from build123d import *

# Parameters (mm, degrees)
PAD023_DEPTH    = 13
SKETCH050_R     = 0.85
POCKET025_DEPTH = 5
FILLET008_R     = 1.2
SKETCH061_W     = 3.59
SKETCH061_H     = 1.95
PAD032_DEPTH    = 1.5
FILLET011_R     = 1


with BuildPart() as part:
    # Sketch049 → Pad023 (new body)
    with BuildSketch(Plane.XZ.offset(-4)):
        Polygon((24.862594, 8.175321), (27.662594, 8.175321), (27.662594, 7.975321), (31.362594, 7.975321), (31.362594, 6.775321), (24.862594, 6.775321), align=None)
    extrude(amount=PAD023_DEPTH)

    # Sketch050 (on Face5 of Pad023) → Pocket025 (cut)
    with BuildSketch(Plane(origin=(0, 0, 6.775321), x_dir=(1, 0, 0), z_dir=(0, 0, -1))):
        with Locations((29.62, 4.4)):
            Circle(SKETCH050_R)
        with Locations((29.62, 0.4)):
            Circle(SKETCH050_R)
    extrude(amount=-POCKET025_DEPTH, mode=Mode.SUBTRACT)

    # Fillet008
    fillet008_edges = [part.edges().sort_by_distance(p)[0] for p in [
        (24.862594, -9, 7.475321),
        (24.862594, 4, 7.475321),
    ]]
    fillet(fillet008_edges, radius=FILLET008_R)

    # Sketch061 (on Face9 of Fillet008) → Pad032 (join)
    with BuildSketch(Plane(origin=(0, 0, 7.975321), x_dir=(-1, 0, 0), z_dir=(0, 0, 1))):
        with Locations((-29.547098, 7.987892)):
            Rectangle(SKETCH061_W, SKETCH061_H)
        with Locations((-29.547098, -2.962108)):
            Rectangle(SKETCH061_W, SKETCH061_H)
    extrude(amount=PAD032_DEPTH)

    # Fillet011
    fillet011_edges = [part.edges().sort_by_distance(p)[0] for p in [
        (27.752098, 2.962108, 9.475321),
        (31.342098, 2.962108, 9.475321),
        (27.752098, -7.987892, 9.475321),
        (31.342098, -7.987892, 9.475321),
    ]]
    fillet(fillet011_edges, radius=FILLET011_R)


with BuildPart() as part_1:
    # Body006 placement: moved
    add(part.part.moved(Location((0, -8.6, 0.6))))


solid = part_1.part
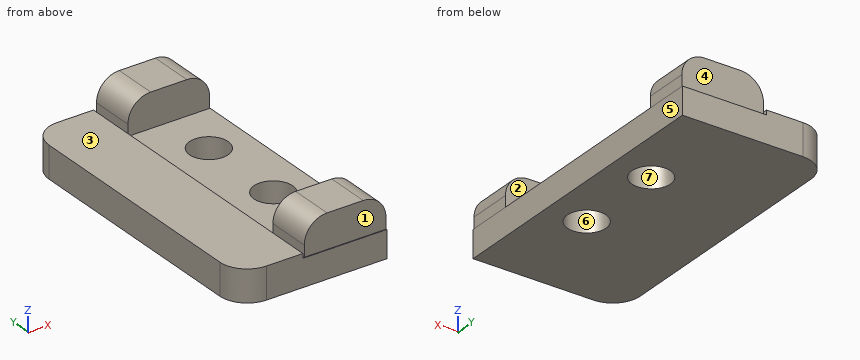
Model file for the job. Use its own axes, mm. Face numbers are marked on the shaded views. A direction names the side the tool comes from. Give positions to 0.01 mm unless a question says otherwise; leave off trailing zeros. Loops run counter-clockwise (first coordinate to the right, second up) from the corner with the lowest first, then second, coordinate; pieces in that order, holes last.
Item 1: Mould opens along X. For the marked faces 4, 5, 6 and 7 say: +X half, -X half, draft (parallel to the pull), parting line (faces both ways), or undercut.
Check values:
face 4: draft
face 5: +X half
face 6: undercut
face 7: undercut
Item 2: Slice it at A-A (y = -13). Write the cut outline in (x, z), plus the area to 3 significant figures.
Check values:
outline: (24.86, 7.38) - (28.77, 7.38) - (28.77, 8.58) - (27.66, 8.58) - (27.66, 8.78) - (24.86, 8.78) - close; (30.47, 7.38) - (31.36, 7.38) - (31.36, 8.58) - (30.47, 8.58) - close
area: 6.32 mm2
Item 3: Drop flat-ended pins along their axis: P1, Ø0.6, axis at y = -17, z = 9, coming from the -X side; P2, Ø0.8, axis at x = 29, z = 9.5, coming from the -Y side; P3, Ø1.4, axis at x = 26.5, y = -11.5, coming from the +Z side. Give the stop position or say it passes through.
Check values:
P1: stops at x = 24.93
P2: stops at y = -17.56
P3: stops at z = 8.78
Item 4: Which spindle directions (+Z, -Z, +X, -X, +Y, -Y) get a long thin tool onto all of the face, cutting with end or side? Do the marked faces 1, 2 and 3. Say none if no direction does.
Check values:
face 1: +Z, +X, -Y
face 2: +Z, +X
face 3: +Z, -X, +Y, -Y
Item 5: Drill centre lines: line 1 along Y through (x, z) = (29.62, 7.7); line 2 along X through (y, z) = (-9, 7.85); line 3 along Y through (x, z) = (29.75, 9.5). Where is each one in solid material? Low to high.
Check values:
line 1: y = -17.6 to -13.85, -12.15 to -9.85, -8.15 to -4.6
line 2: x = 24.86 to 28.77, 30.47 to 31.36
line 3: y = -17.56 to -15.61, -6.61 to -4.66
Item 6: Slice it at B-B (x = 29.62). Give the number of separate pieces and of enclosed holes in the cut face, plus the area to 3 significant figures.
Check values:
separate pieces: 3
enclosed holes: 0
area: 17.4 mm2
Item 7: Slice it at C-C (z = 7.7). Write the cut outline in (x, y), plus the area to 3 significant figures.
Check values:
outline: (24.86, -16.4) arc R1.2 ccw to (26.06, -17.6) - (31.36, -17.6) - (31.36, -4.6) - (26.06, -4.6) arc R1.2 ccw to (24.86, -5.8) - close; hole circle Ø1.7 at (29.62, -13); hole circle Ø1.7 at (29.62, -9)
area: 79.3 mm2
